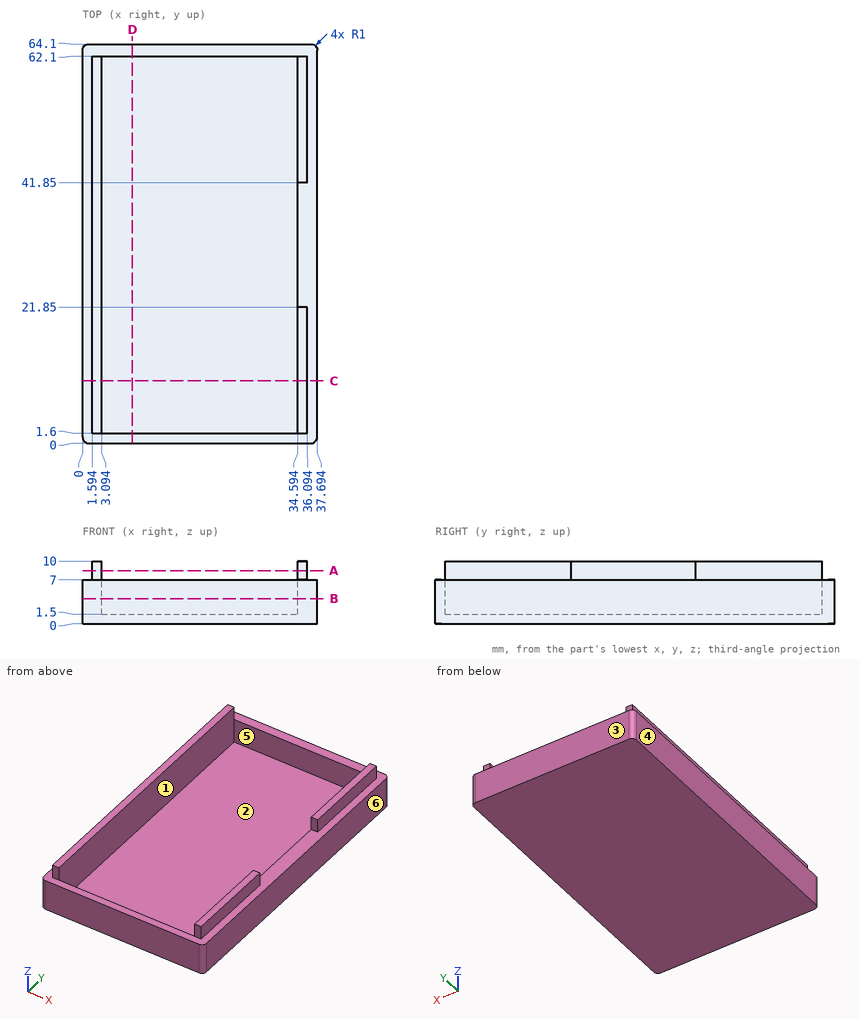
Job drawing, mm, ordinate dimensions from the low corner. One solid piece. A direction names the side the tool comes from. Coordinates: 2 decimals unless noted, no trailing zeros. Order: outer loops, then holes, each group sorted by start corner. A loop starts at its lowest first (then second) coordinate and runs counter-clockwise, first axis right, second up. Notation, with made-up numbers: (61.5, 85) -> (120.5, 85) arc R5 ccw to (120.5, 92) -> close; hole circle Ø6 at (-26.75, 16). An arc over 180 degrees is marked (long way). Return JSON: item names as keys, results as strings. Group by question number.
Item 1: Pull direction Y, two halves, no side cores. Call the marked faces 1, 2, 3 and 4: pulls with the +Y half, pulls with the -Y half, needs draft (parallel to the pull), parting line crosses it, or undercut.
Item 2: Saw through at D-D on x = 8. Write the cut outline in (y, z), then the cut area to 3 significant figures.
Item 3: Saw through at C-C on y = 10. Write the cut outline in (x, z).
Item 4: Flat gauge pins, fed straight in: P1, Ø0.8, axis at x = 35, z = 8.5, coming from the +Y side; P2, Ø2.5, axis at y = 51, z = 8.5, coming from the +X side; P3, Ø1.6, axis at x = 35, z = 9, coming from the -Y side. Where does each tip first touch, or does it go through?
Item 5: Saw through at A-A on z = 8.5. Write the cut outline in (x, y).
Item 6: Saw through at B-B on z = 4. Write the cut outline in (x, y).
Item 7: Tool access for the marked faces 5 and 6: list every direction of +Z, -Z, +X, -X, +Y, -Y with a clear straight run to the whole face (end or side of a thin tool).
Item 8: Wall check: line 1 along X through (y, z) = (8, 4); line 2 along X through (y, z) = (9, 8.5); line 3 along Y through (x, z) = (26, 5.25). Give the ranges that are in metal, low to high. Write a range as [from, to].
Values found:
{
 "1": {"face 1": "undercut", "face 2": "undercut", "face 3": "pulls with the +Y half", "face 4": "needs draft"},
 "2": {"outline": "(0, 0) -> (64.1, 0) -> (64.1, 7) -> (62.1, 7) -> (62.1, 1.5) -> (1.6, 1.5) -> (1.6, 7) -> (0, 7) -> close", "area": "116 mm2"},
 "3": {"outline": "(0, 0) -> (37.69, 0) -> (37.69, 7) -> (36.09, 7) -> (36.09, 10) -> (34.59, 10) -> (34.59, 1.5) -> (3.09, 1.5) -> (3.09, 10) -> (1.59, 10) -> (1.59, 7) -> (0, 7) -> close"},
 "4": {"P1": "stops at y = 62.1", "P2": "stops at x = 36.09", "P3": "stops at y = 1.6"},
 "5": {"outline": "(1.59, 1.6) -> (3.09, 1.6) -> (3.09, 62.1) -> (1.59, 62.1) -> close; (34.59, 1.6) -> (36.09, 1.6) -> (36.09, 21.85) -> (34.59, 21.85) -> close; (34.59, 41.85) -> (36.09, 41.85) -> (36.09, 62.1) -> (34.59, 62.1) -> close"},
 "6": {"outline": "(0, 1) arc R1 ccw to (1, 0) -> (36.69, 0) arc R1 ccw to (37.69, 1) -> (37.69, 63.1) arc R1 ccw to (36.69, 64.1) -> (1, 64.1) arc R1 ccw to (0, 63.1) -> close; hole (3.09, 1.6) -> (34.59, 1.6) -> (34.59, 62.1) -> (3.09, 62.1) -> close"},
 "7": {"face 5": "+Z", "face 6": "+Z, -Z, +X, +Y, -Y"},
 "8": {"line 1": "x = [0, 3.09], [34.59, 37.69]", "line 2": "x = [1.59, 3.09], [34.59, 36.09]", "line 3": "y = [0, 1.6], [62.1, 64.1]"}
}
